Here's how the part is built. I have some questions about the finished solid (model axes, mm). Face numbers are marked on the shaded views. A direction names the side the tool comes from. Round coordinates to 2 decimals unless told otherwise and drop trailing zeros. Loops run counter-clockwise (first coordinate to the right, second up) from the corner with the lowest first, then second, coordinate; pieces in that order, holes last. Notation, with made-up numbers: M -35.5,45 L 2.5,45 A19 cw 2.5,53 Z; hole C -6.5,-24 d5. An arc over 180 degrees is marked long. Write each question's results on one line, items separated by ' | '. Start each with the question number.
```python
from build123d import *

# Parameters (mm, degrees)
F1_DEPTH = 121
F2_T     = -2.54
F4_D     = 6.35


with BuildPart() as f1:
    # F0 (on Front) → F1 (new body, symmetric)
    with BuildSketch(Plane.XZ):
        with BuildLine():
            Line((30.46076, 60.820436), (-2.648024, 60.820436))
            ThreePointArc((-2.648024, 60.820436), (-20.608536, 53.380948), (-28.048024, 35.420436))
            Line((-28.048024, 35.420436), (-28.048024, -44.579564))
            Line((-28.048024, -44.579564), (30.46076, -44.579564))
            Line((30.46076, -44.579564), (30.46076, 60.820436))
        make_face()
    extrude(amount=F1_DEPTH, both=True)

    # F2
    f2_openings = [f1.faces().sort_by_distance(p)[0] for p in [
        (30.46076, 0, 8.120436),
        (1.206368, 0, -44.579564),
    ]]
    offset(amount=F2_T, openings=f2_openings)

    # F4 (through all)
    with Locations(Plane.XZ.offset(121)):
        with Locations((17.797152, -36.322009)):
            Hole(F4_D / 2)


solid = f1.part
```
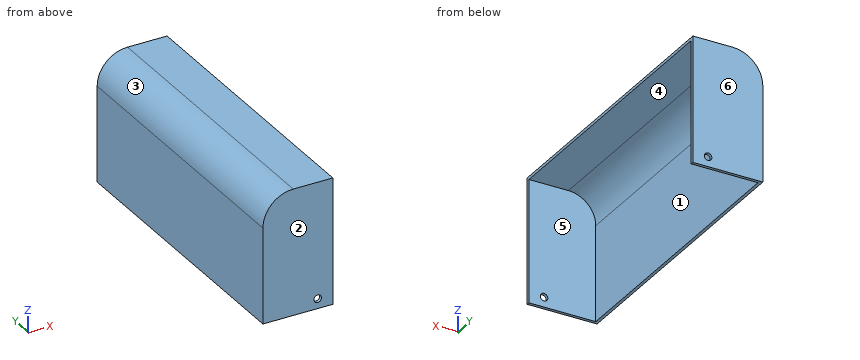
1. I want a section at B-B on y = 61.5. List the corners of the cut face in (x, z) for me.
2. Which directions (+Z, -Z, +X, -X, +Y, -Y) give clear straight access to the entire face, cutting with the end or side of a thin tool? Please do the marked faces 1 and 2.
3. I want a section at A-A on z = -19.5. List the corners of the cut face in (x, y) for me.
4. I need wall thicknesses on line 1 along Y through (x, z) = (27.5, -11.5); line 2 along X through (y, z) = (31.5, -28.5); line 3 along Z through (x, y) = (14, 106.5). Which ranges of each line are inside material? Lowest first, please.
5. If we mould it in two halves opening along Y, with no side actions, what happens to the marked faces 3, 4, 5 and 6? For each: released by +Y, released by -Y, zero draft, split by the parting line, or undercut.
6. For pin 1 (3 mm diameter, centred on y = -51, z = -24, fed in from +X); pin 2 (16.5 mm diameter, centred on x = 11, y = -9, fed in from -Z); pin 3 (2 mm diameter, centred on y = -64, z = 38.5, fed in from -X), each with a flat end and sliding along its axis, tell me the tip position at first contact or that it passes through.
Outcome:
1) outline: M -28.05,-44.58 L -25.51,-44.58 L -25.51,35.42 A22.86 cw -2.65,58.28 L 30.46,58.28 L 30.46,60.82 L -2.65,60.82 A25.4 ccw -28.05,35.42 Z
2) face 1: -Z, +X | face 2: +Z, -Z, +X, -X, -Y
3) outline: M -28.05,-121 L 30.46,-121 L 30.46,-118.46 L -25.51,-118.46 L -25.51,118.46 L 30.46,118.46 L 30.46,121 L -28.05,121 Z
4) line 1: -121 to -118.46, 118.46 to 121 | line 2: -28.05 to -25.51 | line 3: 58.28 to 60.82
5) face 3: zero draft | face 4: undercut | face 5: undercut | face 6: released by +Y
6) pin 1: x = -25.51 | pin 2: z = 58.28 | pin 3: x = -27.96
